Verification items for the finished model (mm, model axes). Face numbers are marked on the shaded views. A direction names the side the tool comes from. Round coordinates to 2 decimals unless told otherwise and drop trailing zeros. Order: outer loops, then holes, each group sorted by start corner. A loop starts at its lowest first (then second) coordinate and runs counter-clockwise, first axis right, second up. Notation, with made-up numbers: (72.5, -22.75) -> (128.5, -22.75) arc R5 ccw to (128.5, -18.75) -> close; hole circle Ø5 at (-11.5, -6). An arc over 180 degrees is marked (long way). Return JSON: item names as keys, results as strings. Group by question number.
1) Draft check along X on the marked faces 6, 7 and 8. Enter one of: pulls with the +X half, pulls with the -X half, needs draft (parallel to the pull), parting line crosses it, or undercut.
2) Section check C-C on y = 25. Enter the section's corners in (x, z).
3) Depth check by flat-ended pin: pin 1 (15 mm diameter, centred on y = 14, z = 7.5, fed in from -X); pin 2 (13 mm diameter, centred on y = 18, z = 0, fed in from +X); pin 3 (18.5 mm diameter, centred on x = 14.5, z = 1.5, fed in from +Y). Enter the tip coordinate at first touch or a pass-through.
4) Section check B-B on x = 11. Enter the section's corners in (y, z).
5) Section check D-D on y = 18. Enter the section's corners in (x, z), plus the area to 3 significant figures.
6) Scan lines: L1, parallel to X at y = 2.8, z = -15; L2, parallel to Z at x = 11, y = 5.45; L3, parallel to X at y = 17.5, z = -13. Record each from-to range of solid material in increasing order.
7) Section check A-A on z = 0. Enter the section's corners in (x, y), plus the area to 3 significant figures.
8) Tool access check on the marked faces 1, 2, 3, 4 and 5. Record the directions out of +Z, -Z, +X, -X, +Y, -Y that give a thin tool (end or side, any length) a straight path to the whole face; none if there is none.
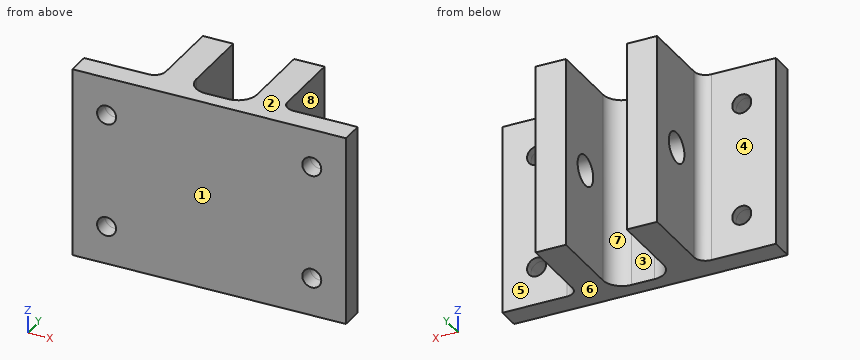
```python
from build123d import *

# Parameters (mm, degrees)
BOSS_EXTRUDE1_DEPTH     = 25
SKETCH2_R               = 4
CUT_EXTRUDE1_DEPTH      = 45
CUT_EXTRUDE1_DEPTH_BACK = 29
FILLET1_R               = 3
FILLET2_R               = 5
SKETCH3_R               = 2.5
CUT_EXTRUDE2_DEPTH      = 25
CUT_EXTRUDE2_DEPTH_BACK = 5


with BuildPart() as part:
    # Sketch1 → Boss-Extrude1 (new body, symmetric)
    with BuildSketch(Plane.XY):
        Polygon((0, 28), (-8, 28), (-8, 4), (-24, 4), (-24, 28), (-32, 28), (-32, 6), (-52, 6), (-52, 0), (-32, 0), (0, 0), (20, 0), (20, 6), (0, 6), align=None)
    extrude(amount=BOSS_EXTRUDE1_DEPTH, both=True)

    # Sketch2 → Cut-Extrude1 (cut, two sides)
    with BuildSketch(Plane.ZY.offset(8)) as cut_extrude1_sk:
        with Locations((0, 18)):
            Circle(SKETCH2_R)
    extrude(amount=CUT_EXTRUDE1_DEPTH, mode=Mode.SUBTRACT)
    extrude(cut_extrude1_sk.sketch, amount=-CUT_EXTRUDE1_DEPTH_BACK, mode=Mode.SUBTRACT)

    # Fillet1
    fillet1_edges = [part.edges().sort_by_distance(p)[0] for p in [
        (0, 6, 0),
        (-32, 6, 0),
    ]]
    fillet(fillet1_edges, radius=FILLET1_R)

    # Fillet2
    fillet2_edges = [part.edges().sort_by_distance(p)[0] for p in [
        (-8, 4, 0),
        (-24, 4, 0),
    ]]
    fillet(fillet2_edges, radius=FILLET2_R)

    # Sketch3 → Cut-Extrude2 (cut, two sides)
    with BuildSketch(Plane(origin=(0, 4, 0), x_dir=(1, 0, 0), z_dir=(0, 1, 0))) as cut_extrude2_sk:
        with Locations((-43, 15)):
            Circle(SKETCH3_R)
        with Locations((11, 15)):
            Circle(SKETCH3_R)
        with Locations((11, -15)):
            Circle(SKETCH3_R)
        with Locations((-43, -15)):
            Circle(SKETCH3_R)
    extrude(amount=CUT_EXTRUDE2_DEPTH, mode=Mode.SUBTRACT)
    extrude(cut_extrude2_sk.sketch, amount=-CUT_EXTRUDE2_DEPTH_BACK, mode=Mode.SUBTRACT)


solid = part.part
```
Check result:
{
 "1": {"face 6": "needs draft", "face 7": "undercut", "face 8": "pulls with the +X half"},
 "2": {"outline": "(-32, -25) -> (-24, -25) -> (-24, 25) -> (-32, 25) -> close; (-8, -25) -> (0, -25) -> (0, 25) -> (-8, 25) -> close"},
 "3": {"pin 1": "x = -33.34", "pin 2": "x = 0", "pin 3": "y = 6"},
 "4": {"outline": "(0, -25) -> (6, -25) -> (6, -17.5) -> (0, -17.5) -> close; (0, -12.5) -> (6, -12.5) -> (6, 12.5) -> (0, 12.5) -> close; (0, 17.5) -> (6, 17.5) -> (6, 25) -> (0, 25) -> close"},
 "5": {"outline": "(-32, -25) -> (-24, -25) -> (-24, -4) -> (-32, -4) -> close; (-32, 4) -> (-24, 4) -> (-24, 25) -> (-32, 25) -> close; (-8, -25) -> (0, -25) -> (0, -4) -> (-8, -4) -> close; (-8, 4) -> (0, 4) -> (0, 25) -> (-8, 25) -> close", "area": "672 mm^2"},
 "6": {"L1": "-52 to -45.5, -40.5 to 8.5, 13.5 to 20", "L2": "-25 to -17.5, -12.5 to 12.5, 17.5 to 25", "L3": "-32 to -24, -8 to 0"},
 "7": {"outline": "(-52, 0) -> (20, 0) -> (20, 6) -> (3, 6) arc R3 cw to (0, 9) -> (0, 14) -> (-8, 14) -> (-8, 9) arc R5 cw to (-13, 4) -> (-19, 4) arc R5 cw to (-24, 9) -> (-24, 14) -> (-32, 14) -> (-32, 9) arc R3 cw to (-35, 6) -> (-52, 6) -> close; (-32, 22) -> (-24, 22) -> (-24, 28) -> (-32, 28) -> close; (-8, 22) -> (0, 22) -> (0, 28) -> (-8, 28) -> close", "area": "639 mm^2"},
 "8": {"face 1": "+Z, -Z, +X, -X, -Y", "face 2": "+Z, +X, -X, +Y, -Y", "face 3": "+Z, -Z, +Y", "face 4": "+Z, -Z, -X, +Y", "face 5": "+Z, -Z, +X, +Y"}
}
